Can you work these out from the model? Positions are in its coordinate system, mm. Round coordinates to 2 decimals unless told otherwise and drop trailing zeros. Order: outer loops, then holes, each group sorted by start corner. A loop starts at its lowest first (then second) coordinate and runs counter-clockwise, first axis right, second up. Notation, with made-up numbers: M -32.5,88 L -19.5,88 A25 cw -19.5,119 Z; hole C 10,-10 d8. An arc over 180 degrees is marked long. One line per question, with ' | ' between items.
```python
from build123d import *

# Parameters (mm, degrees)
F1_DEPTH = 580
F3_DEPTH = 10
F5_DEPTH = 10
F6_R     = 0.5


with BuildPart() as f1:
    # F0 (on Front) → F1 (new body)
    with BuildSketch(Plane.XZ):
        with BuildLine():
            Line((13, -17.5), (13, 7.5))
            ThreePointArc((13, 7.5), (9.1923881554, 16.6923881554), (0, 20.5))
            ThreePointArc((0, 20.5), (-9.1923881554, 16.6923881554), (-13, 7.5))
            Line((-13, 7.5), (-13, -17.5))
            ThreePointArc((-13, -17.5), (-12.1213203436, -19.6213203436), (-10, -20.5))
            Line((-10, -20.5), (10, -20.5))
            ThreePointArc((10, -20.5), (12.1213203436, -19.6213203436), (13, -17.5))
        make_face()
        with BuildLine():
            ThreePointArc((0, 19.5), (8.4852813742, 15.9852813742), (12, 7.5))
            Line((12, 7.5), (12, -10.5))
            Line((12, -10.5), (0, -10.5))
            Line((0, -10.5), (-12, -10.5))
            Line((-12, -10.5), (-12, 7.5))
            ThreePointArc((-12, 7.5), (-8.4852813742, 15.9852813742), (0, 19.5))
        make_face(mode=Mode.SUBTRACT)
        with BuildLine():
            Line((12, -10.5), (12, 7.5))
            ThreePointArc((12, 7.5), (8.4852813742, 15.9852813742), (0, 19.5))
            ThreePointArc((0, 19.5), (-8.4852813742, 15.9852813742), (-12, 7.5))
            Line((-12, 7.5), (-12, -10.5))
            Line((-12, -10.5), (0, -10.5))
            Line((0, -10.5), (12, -10.5))
        make_face()
    extrude(amount=F1_DEPTH)

    # F2 (on face) → F3 (join)
    with BuildSketch(Plane.XZ.offset(580)):
        with BuildLine():
            ThreePointArc((10, -22.5), (13.5355339059, -21.0355339059), (15, -17.5))
            Line((15, -17.5), (15, 7.5))
            ThreePointArc((15, 7.5), (10.6066017178, 18.1066017178), (0, 22.5))
            ThreePointArc((0, 22.5), (-10.6066017178, 18.1066017178), (-15, 7.5))
            Line((-15, 7.5), (-15, -17.5))
            ThreePointArc((-15, -17.5), (-13.5355339059, -21.0355339059), (-10, -22.5))
            Line((-10, -22.5), (10, -22.5))
        make_face()
    extrude(amount=F3_DEPTH)

    # F4 (on face) → F5 (join)
    with BuildSketch(Plane.XZ.offset(590)):
        with BuildLine():
            Line((-12, 7.5), (-12, -10.5))
            Line((-12, -10.5), (0, -10.5))
            Line((0, -10.5), (12, -10.5))
            Line((12, -10.5), (12, 7.5))
            ThreePointArc((12, 7.5), (8.4852813742, 15.9852813742), (0, 19.5))
            ThreePointArc((0, 19.5), (-8.4852813742, 15.9852813742), (-12, 7.5))
        make_face()
    extrude(amount=F5_DEPTH)

    # F6
    f6_edges = [f1.edges().sort_by_distance(p)[0] for p in [
        (0, -600, -10.5),
        (-12, -600, -1.5),
        (-15, -590, -5),
        (0, -590, 22.5),
        (-15, -580, -5),
    ]]
    fillet(f6_edges, radius=F6_R)

    # F7: F1 across plane


with BuildPart() as f1_1:
    add(f1.part)
    add(f1.part.mirror(Plane.XZ))

    # F8: F1 across plane


with BuildPart() as f1_2:
    add(f1_1.part)
    add(f1_1.part.mirror(Plane.XZ))


solid = f1_2.part
```
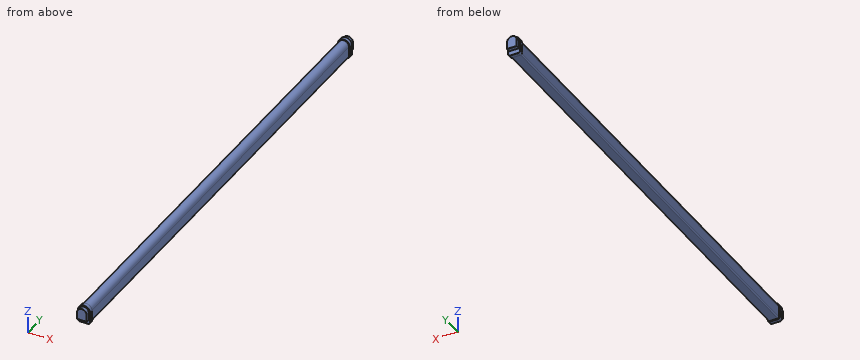
(1) Please list where these lines run through material, in increasing order: probe 1 along Y at (x, z) = (12.5, 12.5); probe 2 along X at (y, z) = (-164.5, 0); probe 3 along Y at (x, z) = (12, -15). Write a range as [from, to].
Final values:
probe 1: [-590, -580], [580, 590] | probe 2: [-13, 13] | probe 3: [-590, 590]
(2) If we section it at A-A on y = 444: Please give me the cut outline in (x, z), plus the area to 3 significant figures.
Final values:
outline: M -13,-17.5 A3 ccw -10,-20.5 L 10,-20.5 A3 ccw 13,-17.5 L 13,7.5 A13 ccw -13,7.5 Z | area: 990 mm^2
(3) Will these pins go through, and if not, where does the flat tip stop? pin 1 Ø12 at (y, z) = (247.5, 16.5) entering from -X; pin 2 Ø7.5 at (x, y) = (-3.5, 594) entering from -Z; pin 3 Ø3 at (y, z) = (-594.5, -0.5) entering from -X.
Final values:
pin 1: x = -12.65 | pin 2: z = -10.5 | pin 3: x = -12
